from build123d import *

# Parameters (mm, degrees)
F1_DEPTH = 25.4
F3_DEPTH = 25.4
F6_DEPTH = 12.7
F7_DEPTH = 12.7


with BuildPart() as f1:
    # F0 (on Top) → F1 (new body)
    with BuildSketch(Plane.XY):
        Polygon((0, 25.4), (0, 0), (12.7, 0), (12.7, 25.4), (25.4, 25.4), (25.4, 44.45), (-12.7, 44.45), (-12.7, 25.4), align=None)
    extrude(amount=F1_DEPTH)

    # F2 (on face) → F3 (cut)
    with BuildSketch(Plane(origin=(0, 0, 0), x_dir=(0, -1, 0), z_dir=(-1, 0, 0))):
        Polygon((-8.356945, 25.4), (0, 0), (0, 25.4), align=None)
    extrude(amount=-F3_DEPTH, mode=Mode.SUBTRACT)

    # F5 (on face) → F6 (cut)
    with BuildSketch(Plane.YZ.offset(25.4)):
        Polygon((25.4, 0), (31.670947, 25.4), (25.4, 25.4), align=None)
    extrude(amount=-F6_DEPTH, mode=Mode.SUBTRACT)

    # F4 (on face) → F7 (cut)
    with BuildSketch(Plane(origin=(-12.7, 0, 0), x_dir=(0, -1, 0), z_dir=(-1, 0, 0))):
        Polygon((-31.880192, 25.4), (-25.4, 0), (-25.4, 25.4), align=None)
    extrude(amount=-F7_DEPTH, mode=Mode.SUBTRACT)


solid = f1.part
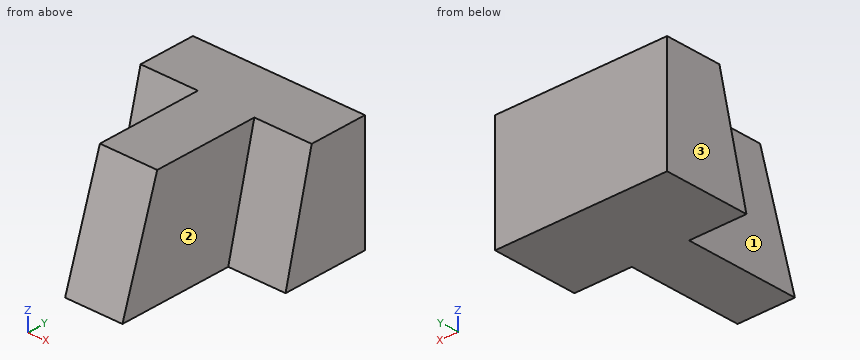
Check sheet for the modelled part. Datum: model origin and axes. Units: mm. Face numbers are marked on the shaded views. A direction names the side the tool comes from. Coordinates: 2 decimals unless noted, no trailing zeros. Loops run counter-clockwise (first coordinate to the right, second up) from the corner with the lowest first, then second, coordinate; pieces in that order, holes last. Notation, with made-up numbers: (9.25, -14) -> (29.25, -14) arc R31 cw to (29.25, 24) -> close; hole circle Ø3 at (26.5, 63). An arc over 180 degrees is marked (long way). Write item = value, one per line. Start each with the question number.
1. Tool access check on the marked faces 1, 2 and 3. Record the directions out of +Z, -Z, +X, -X, +Y, -Y that give a thin tool (end or side, any length) a straight path to the whole face; none if there is none.
2. Section check A-A on z = 19.75. Record the cut outline in (x, y), then the cut area to 3 significant figures.
3. Section check C-C on y = 27. Record the cut outline in (x, z), then the cut area to 3 significant figures.
4. Section check D-D on y = 19. Record the cut outline in (x, z), then the cut area to 3 significant figures.
5. Section check B-B on x = 4.5. Record the cut outline in (y, z), then the cut area to 3 significant figures.
6. Material ranges on line 1 (X direction, y = 8.5, z = 7.5); line 2 (Y direction, x = 8, z = 1.75); line 3 (Y direction, x = -8, z = 21.75), recorded low to high.
7. Depth check by flat-ended pin: P1, Ø5, axis at y = 18.5, z = 8, coming from the -X side; P2, Ø1.5, axis at x = -8.5, z = 4.5, coming from the -Y side. Enter the tip coordinate at first touch or a pass-through.
Responses:
q1.face_1 = +Z, -X, -Y
q1.face_2 = +Z, +X, -Y
q1.face_3 = +Z, -Z, -X, +Y, -Y
q2.outline = (-12.7, 30.44) -> (0, 30.44) -> (0, 6.5) -> (12.7, 6.5) -> (12.7, 30.28) -> (25.4, 30.28) -> (25.4, 44.45) -> (-12.7, 44.45) -> close
q2.area = 840 mm2
q3.outline = (-12.7, 0) -> (25.4, 0) -> (25.4, 6.48) -> (12.7, 6.48) -> (12.7, 25.4) -> (0, 25.4) -> (0, 6.27) -> (-12.7, 6.27) -> close
q3.area = 485 mm2
q4.outline = (0, 0) -> (12.7, 0) -> (12.7, 25.4) -> (0, 25.4) -> close
q4.area = 323 mm2
q5.outline = (0, 0) -> (44.45, 0) -> (44.45, 25.4) -> (8.36, 25.4) -> close
q5.area = 1,020 mm2
q6.line_1 = 0 to 12.7
q6.line_2 = 0.58 to 44.45
q6.line_3 = 30.95 to 44.45
q7.P1 = 0
q7.P2 = 26.36
